Verification items for the finished model (mm, model axes). A direction names the side the tool comes from. Give positions to 0.01 mm unless a question says otherwise; leave off trailing zeros. Loops run counter-clockwise (first coordinate to the right, second up) from the corner with the lowest first, then second, coordinate; pieces in that order, holes last. Notation, with made-up numbers: (87.5, -26.5) -> (125.5, -26.5) arc R24 ccw to (125.5, -12.5) -> close; hole circle Ø1 at (75.5, 88.25). An arc over 180 degrees is marked (long way). Answer in a Markdown table with one row per item. Add a question column.
Q1. Section check B-B on z = 24. Enter the section's corners in (x, y).
Q2. Material ranges on probe 1 along Z at (x, y) = (12, 8.5); probe 2 along X at (y, z) = (63.5, -21.5); probe 3 along Y at (x, z) = (-15, 88), recorded low to high.
Q3. Section check D-D on y = 12.5. Enter the section's corners in (x, z).
Q4. Set-up check for faces 5 (the face through (19, 35, -32)), 6 (the face through (35, 0, 57)), 7 (the face through (-1, 29, -30)), 8 (the face through (-47, 51, 27)): record each of +Z, -Z, +X, -X, +Y, -Y from which the full face is reachable in a straight line by a thin tool's end or side.
Q5. Section check A-A on x = -22. Enter the section's corners in (y, z).
Q6. Release check for a two-part mould opening along Z. For faces 1 (the face through (36.5, 30, -32)), 2 (the face through (47, -5, 5)), 3 (the face through (-47, 51, 9)), 4 (the face through (-47, 52, -26.5)) record: pulls with the +Z half, pulls with the -Z half, needs draft (parallel to the pull), parting line crosses it, or undercut.
Q7. Section check C-C on x = 0. Enter the section's corners in (y, z).
Q8. Gauge pin test, flat ends, axial feed: P1, Ø2.5, axis at y = -6, z = 88.5, coming from the -X side; P2, Ø3.5, axis at y = 29, z = -31, coming from the +X side; P3, Ø1.5, axis at x = 16, z = 89, coming from the -Y side; P4, Ø4, axis at x = 0, y = -5, coming from the +Z side. Record the tip position at first contact, or that the pin passes through.
```python
from build123d import *

# Parameters (mm, degrees)
BOSS_EXTRUDE2_DEPTH            = 69
CHAMFER1_SIZE                  = 3
CHAMFER2_SIZE                  = 5
SKETCH5_W                      = 10
SKETCH5_H                      = 3
SKETCH5_W_2                    = 3
SKETCH5_H_2                    = 10
BOSS_EXTRUDE3_DEPTH            = 10
SKETCH6_R                      = 1.75
CUT_EXTRUDE1_DEPTH             = 150.231363996
SKETCH7_R                      = 1.75
CUT_EXTRUDE2_DEPTH             = 150.13835858
CUT_EXTRUDE3_REACH             = 151.138
SKETCH8_W                      = 57
SKETCH8_H                      = 10
SKETCH8_W_2                    = 35
CUT_EXTRUDE4_REACH             = 151.231
SKETCH10_W                     = 15
SKETCH10_H                     = 18
SKETCH10_W_2                   = 18
SKETCH10_H_2                   = 16
CUT_EXTRUDE5_REACH             = 143.426
SKETCH12_W                     = 12
SKETCH12_H                     = 7
CUT_EXTRUDE5_DIRECTION_2_DEPTH = 142.425775586
CUT_EXTRUDE6_REACH             = 151.231
SKETCH14_R                     = 6
CUT_EXTRUDE7_REACH             = 151.138
SKETCH15_W                     = 13
SKETCH15_H                     = 19
CUT_EXTRUDE8_REACH             = 151.231
SKETCH16_W                     = 14
SKETCH16_H                     = 10
CUT_EXTRUDE9_REACH             = 151.231
SKETCH18_W                     = 7
SKETCH18_H                     = 3
CHAMFER3_SIZE                  = 0.5
CUT_EXTRUDE10_REACH            = 151.138
SKETCH19_R                     = 3.75


with BuildPart() as part:
    # Sketch4 → Boss-Extrude2 (new body)
    with BuildSketch(Plane(origin=(0, 0, 0), x_dir=(1, 0, 0), z_dir=(0, 1, 0))):
        Polygon((-48.5, 33), (48.5, 33), (48.5, -29.22455366), (36, -58.572379747), (36, -90), (-36, -90), (-36, -58.572379747), (-48.5, -29.22455366), align=None)
        Polygon((-45.5, 30), (45.5, 30), (45.5, -28.61227683), (33, -57.960102917), (33, -87), (-33, -87), (-33, -57.960102917), (-45.5, -28.61227683), align=None, mode=Mode.SUBTRACT)
    extrude(amount=BOSS_EXTRUDE2_DEPTH)

    # Chamfer1
    chamfer1_edges = [part.edges().sort_by_distance(p)[0] for p in [
        (-45.5, 34.5, -30),
        (-33, 34.5, 87),
        (33, 34.5, 87),
        (45.5, 34.5, -30),
    ]]
    chamfer(chamfer1_edges, length=CHAMFER1_SIZE)

    # Chamfer2
    chamfer2_edges = [part.edges().sort_by_distance(p)[0] for p in [
        (-48.5, 34.5, -33),
        (48.5, 34.5, -33),
        (36, 34.5, 90),
        (-36, 34.5, 90),
    ]]
    chamfer(chamfer2_edges, length=CHAMFER2_SIZE)

    # Sketch5 → Boss-Extrude3 (add)
    with BuildSketch(Plane(origin=(0, 0, 0), x_dir=(1, 0, 0), z_dir=(0, 1, 0))):
        with Locations((0, 31.5)):
            Rectangle(SKETCH5_W, SKETCH5_H)
        with Locations((-47, 0)):
            Rectangle(SKETCH5_W_2, SKETCH5_H_2)
        with Locations((0, -88.5)):
            Rectangle(SKETCH5_W, SKETCH5_H)
        with Locations((47, 0)):
            Rectangle(SKETCH5_W_2, SKETCH5_H_2)
    extrude(amount=-BOSS_EXTRUDE3_DEPTH)

    # Sketch6 → Cut-Extrude1 (cut, through all)
    with BuildSketch(Plane.ZY.offset(48.5)):
        with Locations((0, -5)):
            Circle(SKETCH6_R)
    extrude(amount=-CUT_EXTRUDE1_DEPTH, mode=Mode.SUBTRACT)

    # Sketch7 → Cut-Extrude2 (cut, through all)
    with BuildSketch(Plane(origin=(0, 0, -33), x_dir=(-1, 0, 0), z_dir=(0, 0, -1))):
        with Locations((0, -5)):
            Circle(SKETCH7_R)
    extrude(amount=-CUT_EXTRUDE2_DEPTH, mode=Mode.SUBTRACT)

    # Sketch8 → Cut-Extrude3 (cut, up to next)
    with BuildSketch(Plane(origin=(0, 0, -33), x_dir=(-1, 0, 0), z_dir=(0, 0, -1)), mode=Mode.PRIVATE) as cut_extrude3_sk1:
        with Locations((-11, 45)):
            Rectangle(SKETCH8_W, SKETCH8_H)
    cut_extrude3_tool1 = extrude(cut_extrude3_sk1.sketch, amount=-CUT_EXTRUDE3_REACH, mode=Mode.PRIVATE) & part.part
    # Sketch8 → Cut-Extrude3 (cut, up to next)
    with BuildSketch(Plane(origin=(0, 0, -33), x_dir=(-1, 0, 0), z_dir=(0, 0, -1)), mode=Mode.PRIVATE) as cut_extrude3_sk2:
        with Locations((-19, 30)):
            Rectangle(SKETCH8_W_2, SKETCH8_H)
    cut_extrude3_tool2 = extrude(cut_extrude3_sk2.sketch, amount=-CUT_EXTRUDE3_REACH, mode=Mode.PRIVATE) & part.part
    add(cut_extrude3_tool1.solids().sort_by_distance((11, 45, -33))[0], mode=Mode.SUBTRACT)
    add(cut_extrude3_tool2.solids().sort_by_distance((19, 30, -33))[0], mode=Mode.SUBTRACT)

    # Sketch10 → Cut-Extrude4 (cut, up to next)
    with BuildSketch(Plane.ZY.offset(48.5), mode=Mode.PRIVATE) as cut_extrude4_sk1:
        with Locations((-19, 52)):
            Rectangle(SKETCH10_W, SKETCH10_H)
    cut_extrude4_tool1 = extrude(cut_extrude4_sk1.sketch, amount=-CUT_EXTRUDE4_REACH, mode=Mode.PRIVATE) & part.part
    # Sketch10 → Cut-Extrude4 (cut, up to next)
    with BuildSketch(Plane.ZY.offset(48.5), mode=Mode.PRIVATE) as cut_extrude4_sk2:
        with Locations((-1, 52)):
            Rectangle(SKETCH10_W, SKETCH10_H)
    cut_extrude4_tool2 = extrude(cut_extrude4_sk2.sketch, amount=-CUT_EXTRUDE4_REACH, mode=Mode.PRIVATE) & part.part
    # Sketch10 → Cut-Extrude4 (cut, up to next)
    with BuildSketch(Plane.ZY.offset(48.5), mode=Mode.PRIVATE) as cut_extrude4_sk3:
        with Locations((18, 51)):
            Rectangle(SKETCH10_W_2, SKETCH10_H_2)
    cut_extrude4_tool3 = extrude(cut_extrude4_sk3.sketch, amount=-CUT_EXTRUDE4_REACH, mode=Mode.PRIVATE) & part.part
    add(cut_extrude4_tool1.solids().sort_by_distance((-48.5, 52, -19))[0], mode=Mode.SUBTRACT)
    add(cut_extrude4_tool2.solids().sort_by_distance((-48.5, 52, -1))[0], mode=Mode.SUBTRACT)
    add(cut_extrude4_tool3.solids().sort_by_distance((-48.5, 51, 18))[0], mode=Mode.SUBTRACT)

    # Sketch12 → Cut-Extrude5 (cut, up to next)
    with BuildSketch(Plane.ZY.offset(36), mode=Mode.PRIVATE) as cut_extrude5_sk1:
        with Locations((64.072379747, 43.5)):
            Rectangle(SKETCH12_W, SKETCH12_H)
    cut_extrude5_tool1 = extrude(cut_extrude5_sk1.sketch, amount=-CUT_EXTRUDE5_REACH, mode=Mode.PRIVATE) & part.part
    add(cut_extrude5_tool1.solids().sort_by_distance((-36, 43.5, 64.07238))[0], mode=Mode.SUBTRACT)

    # Sketch12 → Cut-Extrude5 direction 2 (cut)
    with BuildSketch(Plane.ZY.offset(36)):
        with Locations((64.072379747, 43.5)):
            Rectangle(SKETCH12_W, SKETCH12_H)
    extrude(amount=CUT_EXTRUDE5_DIRECTION_2_DEPTH, mode=Mode.SUBTRACT)

    # Sketch14 → Cut-Extrude6 (cut, up to next)
    with BuildSketch(Plane(origin=(48.5, 0, 0), x_dir=(0, 0, -1), z_dir=(1, 0, 0)), mode=Mode.PRIVATE) as cut_extrude6_sk1:
        with Locations((-5, 56)):
            Circle(SKETCH14_R)
    cut_extrude6_tool1 = extrude(cut_extrude6_sk1.sketch, amount=-CUT_EXTRUDE6_REACH, mode=Mode.PRIVATE) & part.part
    add(cut_extrude6_tool1.solids().sort_by_distance((48.5, 56, 5))[0], mode=Mode.SUBTRACT)

    # Sketch15 → Cut-Extrude7 (cut, up to next)
    with BuildSketch(Plane.XY.offset(90), mode=Mode.PRIVATE) as cut_extrude7_sk1:
        with Locations((16.5, 19.5)):
            Rectangle(SKETCH15_W, SKETCH15_H)
    cut_extrude7_tool1 = extrude(cut_extrude7_sk1.sketch, amount=-CUT_EXTRUDE7_REACH, mode=Mode.PRIVATE) & part.part
    add(cut_extrude7_tool1.solids().sort_by_distance((16.5, 19.5, 90))[0], mode=Mode.SUBTRACT)

    # Sketch16 → Cut-Extrude8 (cut, up to next)
    with BuildSketch(Plane(origin=(48.5, 0, 0), x_dir=(0, 0, -1), z_dir=(1, 0, 0)), mode=Mode.PRIVATE) as cut_extrude8_sk1:
        with Locations((-0.5, 38)):
            Rectangle(SKETCH16_W, SKETCH16_H)
    cut_extrude8_tool1 = extrude(cut_extrude8_sk1.sketch, amount=-CUT_EXTRUDE8_REACH, mode=Mode.PRIVATE) & part.part
    add(cut_extrude8_tool1.solids().sort_by_distance((48.5, 38, 0.5))[0], mode=Mode.SUBTRACT)

    # Sketch18 → Cut-Extrude9 (cut, up to next)
    with BuildSketch(Plane(origin=(48.5, 0, 0), x_dir=(0, 0, -1), z_dir=(1, 0, 0)), mode=Mode.PRIVATE) as cut_extrude9_sk1:
        with Locations((18.5, 44.5)):
            Rectangle(SKETCH18_W, SKETCH18_H)
    cut_extrude9_tool1 = extrude(cut_extrude9_sk1.sketch, amount=-CUT_EXTRUDE9_REACH, mode=Mode.PRIVATE) & part.part
    add(cut_extrude9_tool1.solids().sort_by_distance((48.5, 44.5, -18.5))[0], mode=Mode.SUBTRACT)

    # Chamfer3
    chamfer3_edges = [part.edges().sort_by_distance(p)[0] for p in [
        (-39.25, 69, 43.286189873),
        (-33, 69, 70.980051458),
        (39.25, 69, 43.286189873),
        (45.5, 69, 0.806138415),
        (0, 69, 87),
        (33, 69, 70.980051458),
        (0, 69, -30),
        (-45.5, 69, 0.806138415),
        (-31.5, 69, 85.5),
        (31.5, 69, 85.5),
        (44, 69, -28.5),
        (-44, 69, -28.5),
    ]]
    chamfer(chamfer3_edges, length=CHAMFER3_SIZE)

    # Sketch19 → Cut-Extrude10 (cut, up to next)
    with BuildSketch(Plane.XY.offset(90), mode=Mode.PRIVATE) as cut_extrude10_sk1:
        with Locations((-15, 19.5)):
            Circle(SKETCH19_R)
    cut_extrude10_tool1 = extrude(cut_extrude10_sk1.sketch, amount=-CUT_EXTRUDE10_REACH, mode=Mode.PRIVATE) & part.part
    add(cut_extrude10_tool1.solids().sort_by_distance((-15, 19.5, 90))[0], mode=Mode.SUBTRACT)


solid = part.part
```
Taken from the geometry:
| question | item | result |
|---|---|---|
| 1 | outline | (-48.5, 0) -> (-45.5, 0) -> (-45.5, 43) -> (-48.5, 43) -> close; (-48.5, 59) -> (-45.5, 59) -> (-45.5, 68.5) -> (-46, 69) -> (-48.5, 69) -> close; (45.5, 0) -> (48.5, 0) -> (48.5, 69) -> (46, 69) -> (45.5, 68.5) -> close |
| 2 | probe 1 | z = -33 to -30, 87 to 90 |
| 2 | probe 2 | x = -48.5 to -45.5, 45.5 to 48.5 |
| 2 | probe 3 | y = 0 to 15.75, 23.25 to 69 |
| 3 | outline | (-48.5, -28) -> (-43.5, -33) -> (43.5, -33) -> (48.5, -28) -> (48.5, 29.22) -> (36, 58.57) -> (36, 85) -> (31, 90) -> (23, 90) -> (23, 87) -> (30, 87) -> (33, 84) -> (33, 57.96) -> (45.5, 28.61) -> (45.5, -27) -> (42.5, -30) -> (-42.5, -30) -> (-45.5, -27) -> (-45.5, 28.61) -> (-33, 57.96) -> (-33, 84) -> (-30, 87) -> (10, 87) -> (10, 90) -> (-31, 90) -> (-36, 85) -> (-36, 58.57) -> (-48.5, 29.22) -> close |
| 4 | face 5 | -Z |
| 4 | face 6 | +Z, +X, -Y |
| 4 | face 7 | +Y, -Y |
| 4 | face 8 | -X |
| 5 | outline | (0, -33) -> (69, -33) -> (69, -30.5) -> (68.5, -30) -> (0, -30) -> close; (0, 87) -> (68.5, 87) -> (69, 87.5) -> (69, 90) -> (0, 90) -> close |
| 6 | face 1 | needs draft |
| 6 | face 2 | pulls with the +Z half |
| 6 | face 3 | undercut |
| 6 | face 4 | undercut |
| 7 | outline | (-10, -33) -> (-6.75, -33) -> (-6.75, -30) -> (-10, -30) -> close; (-10, 87) -> (-6.75, 87) -> (-6.75, 90) -> (-10, 90) -> close; (-3.25, -33) -> (40, -33) -> (40, -30) -> (-3.25, -30) -> close; (-3.25, 87) -> (68.5, 87) -> (69, 87.5) -> (69, 90) -> (-3.25, 90) -> close; (50, -33) -> (69, -33) -> (69, -30.5) -> (68.5, -30) -> (50, -30) -> close |
| 8 | P1 | stops at x = -5 |
| 8 | P2 | stops at x = 47.25 |
| 8 | P3 | stops at y = 0 |
| 8 | P4 | stops at z = 90 |
